```python
from build123d import *

# Parameters (mm, degrees)
BOSS_EXTRUDE1_DEPTH = 4
BOSS_EXTRUDE1_TAPER = 10
CUT_EXTRUDE1_START  = 4
SKETCH1_3_R         = 1.1
CUT_EXTRUDE1_DEPTH  = 4
CUT_EXTRUDE2_START  = 4
SKETCH1_4_R         = 8.4
SKETCH1_4_R_2       = 1.1
CUT_EXTRUDE2_DEPTH  = 3


with BuildPart() as part:
    # Sketch1 → Boss-Extrude1 (new body)
    with BuildSketch(Plane(origin=(0, 0, 0), x_dir=(1, 0, 0), z_dir=(0, 1, 0))):
        with BuildLine():
            Line((-49.472689603, -5.7), (-39.572689603, -22.847302995))
            ThreePointArc((-39.572689603, -22.847302995), (-35.4, -27.019992598), (-29.7, -28.547302995))
            Line((-29.7, -28.547302995), (-9.9, -28.547302995))
            ThreePointArc((-9.9, -28.547302995), (-4.2, -27.019992598), (-0.027310397, -22.847302995))
            Line((-0.027310397, -22.847302995), (9.872689603, -5.7))
            ThreePointArc((9.872689603, -5.7), (9.872689603, 5.7), (0, 11.4))
            Line((0, 11.4), (-39.6, 11.4))
            ThreePointArc((-39.6, 11.4), (-49.472689603, 5.7), (-49.472689603, -5.7))
        make_face()
    extrude(amount=BOSS_EXTRUDE1_DEPTH, taper=BOSS_EXTRUDE1_TAPER)

    # Sketch1<3> → Cut-Extrude1 (cut)
    with BuildSketch(Plane(origin=(0, 0, 0), x_dir=(1, 0, 0), z_dir=(0, 1, 0)).offset(CUT_EXTRUDE1_START)):
        with Locations(Location((-9.9, -17.147302995, 0), (0, 0, 270))):
            Circle(SKETCH1_3_R)
        with Locations(Location((0, 0, 0), (0, 0, 270))):
            Circle(SKETCH1_3_R)
        with Locations(Location((-29.7, -17.147302995, 0), (0, 0, 270))):
            Circle(SKETCH1_3_R)
        with Locations(Location((-39.6, 0, 0), (0, 0, 270))):
            Circle(SKETCH1_3_R)
        with Locations(Location((-19.8, 0, 0), (0, 0, 270))):
            Circle(SKETCH1_3_R)
    extrude(amount=-CUT_EXTRUDE1_DEPTH, mode=Mode.SUBTRACT)

    # Sketch1<4> → Cut-Extrude2 (cut)
    # profile 1 of 5: a face of its own
    with BuildSketch(Plane(origin=(0, 0, 0), x_dir=(1, 0, 0), z_dir=(0, 1, 0)).offset(CUT_EXTRUDE2_START)):
        with Locations(Location((-19.8, 0, 0), (0, 0, 270))):
            Circle(SKETCH1_4_R)
        with Locations(Location((-19.8, 0, 0), (0, 0, 270))):
            Circle(SKETCH1_4_R_2, mode=Mode.SUBTRACT)
    # profile 2 of 5: a face of its own
    with BuildSketch(Plane(origin=(0, 0, 0), x_dir=(1, 0, 0), z_dir=(0, 1, 0)).offset(CUT_EXTRUDE2_START)):
        with Locations(Location((-9.9, -17.147302995, 0), (0, 0, 270))):
            Circle(SKETCH1_4_R)
        with Locations(Location((-9.9, -17.147302995, 0), (0, 0, 270))):
            Circle(SKETCH1_4_R_2, mode=Mode.SUBTRACT)
    # profile 3 of 5: a face of its own
    with BuildSketch(Plane(origin=(0, 0, 0), x_dir=(1, 0, 0), z_dir=(0, 1, 0)).offset(CUT_EXTRUDE2_START)):
        with Locations(Location((0, 0, 0), (0, 0, 270))):
            Circle(SKETCH1_4_R)
        with Locations(Location((0, 0, 0), (0, 0, 270))):
            Circle(SKETCH1_4_R_2, mode=Mode.SUBTRACT)
    # profile 4 of 5: a face of its own
    with BuildSketch(Plane(origin=(0, 0, 0), x_dir=(1, 0, 0), z_dir=(0, 1, 0)).offset(CUT_EXTRUDE2_START)):
        with Locations(Location((-29.7, -17.147302995, 0), (0, 0, 270))):
            Circle(SKETCH1_4_R)
        with Locations(Location((-29.7, -17.147302995, 0), (0, 0, 270))):
            Circle(SKETCH1_4_R_2, mode=Mode.SUBTRACT)
    # profile 5 of 5: a face of its own
    with BuildSketch(Plane(origin=(0, 0, 0), x_dir=(1, 0, 0), z_dir=(0, 1, 0)).offset(CUT_EXTRUDE2_START)):
        with Locations(Location((-39.6, 0, 0), (0, 0, 270))):
            Circle(SKETCH1_4_R)
        with Locations(Location((-39.6, 0, 0), (0, 0, 270))):
            Circle(SKETCH1_4_R_2, mode=Mode.SUBTRACT)
    extrude(amount=-CUT_EXTRUDE2_DEPTH, mode=Mode.SUBTRACT)


solid = part.part
```
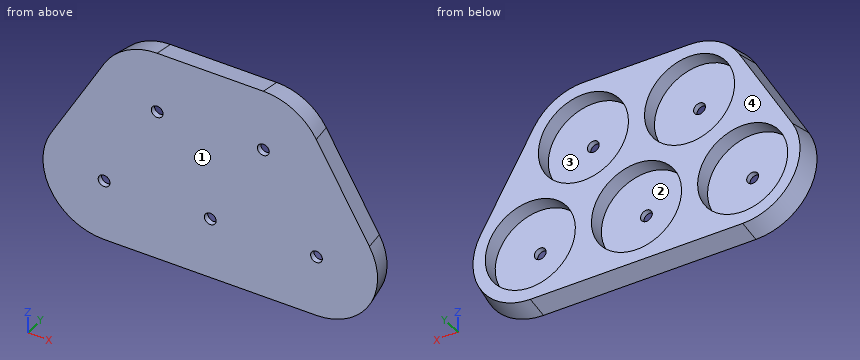
Here's how the part is built. I have some questions about the finished solid (model axes, mm). Face numbers are marked on the shaded views. A direction names the side the tool comes from. Round coordinates to 2 decimals unless told otherwise and drop trailing zeros. One line per question, with ' | ' between items.
1) For pin 1 Ø3.5 at (x, z) = (0, 0) entering from +Y; pin 2 Ø6 at (x, z) = (-40, 11) entering from -Y; pin 3 Ø2 at (x, y) = (-14, 2) entering from -Z; pin 4 Ø1 at (y, z) = (1, 6.5) entering from +X, each with a flat end and sliding along its axis, tell me the tip position at first contact or that it passes through.
Working result:
pin 1: y = 1 | pin 2: y = 0 | pin 3: z = -11.22 | pin 4: x = 9.51
2) For the marked faces 3 and 4, which set-ups out of +Z, -Z, +X, -X, +Y, -Y let a thin tool reach every point of the face, with its end or its side?
Working result:
face 3: +Y | face 4: +Z, -Z, +X, -X, +Y
3) I want a section at A-A, the plane z = 0. State how many separate pieces and enclosed holes the cut face has, then the cut area to 3 significant figures.
Working result:
separate pieces: 4 | enclosed holes: 0 | area: 89.0 mm²
4) I need wall thicknesses on line 1 along X through (y, z) = (1.1, 19.5); line 2 along X through (y, z) = (3.1, -4.5); line 3 along Z through (x, y) = (-23, 3.1). Which ranges of each line are inside material? Lowest first, please.
Working result:
line 1: -41.28 to -37.76, -21.64 to -17.96, -1.84 to 1.68 | line 2: -49.48 to -46.69, -32.51 to -26.89, -12.71 to -7.09, 7.09 to 9.88 | line 3: -10.85 to -7.77, 7.77 to 12.08, 22.21 to 28
5) If we mould it in two halves opening along X, with no side actions, what happens to the marked faces 1 and 2? For each: +X half, -X half, draft (parallel to the pull), parting line (faces both ways), or undercut.
Working result:
face 1: draft | face 2: undercut
